Drawing for the job (mm, zero at the part's lowest x, y, z). Round coordinates to 2 decimals unless told otherwise and drop trailing zeros. Order: outer loops, then holes, each group sorted by start corner. A loop starts at its lowest first (then second) coordinate and runs counter-clockwise, first axis right, second up. Notation, with made-up numbers: (22.25, 33) -> (36.25, 33) arc R3 cw to (36.25, 37) -> close; hole circle Ø2 at (-23.75, -30). An arc over 180 degrees is marked (long way). Answer as CSV lines item,"result". Start each with the question number.
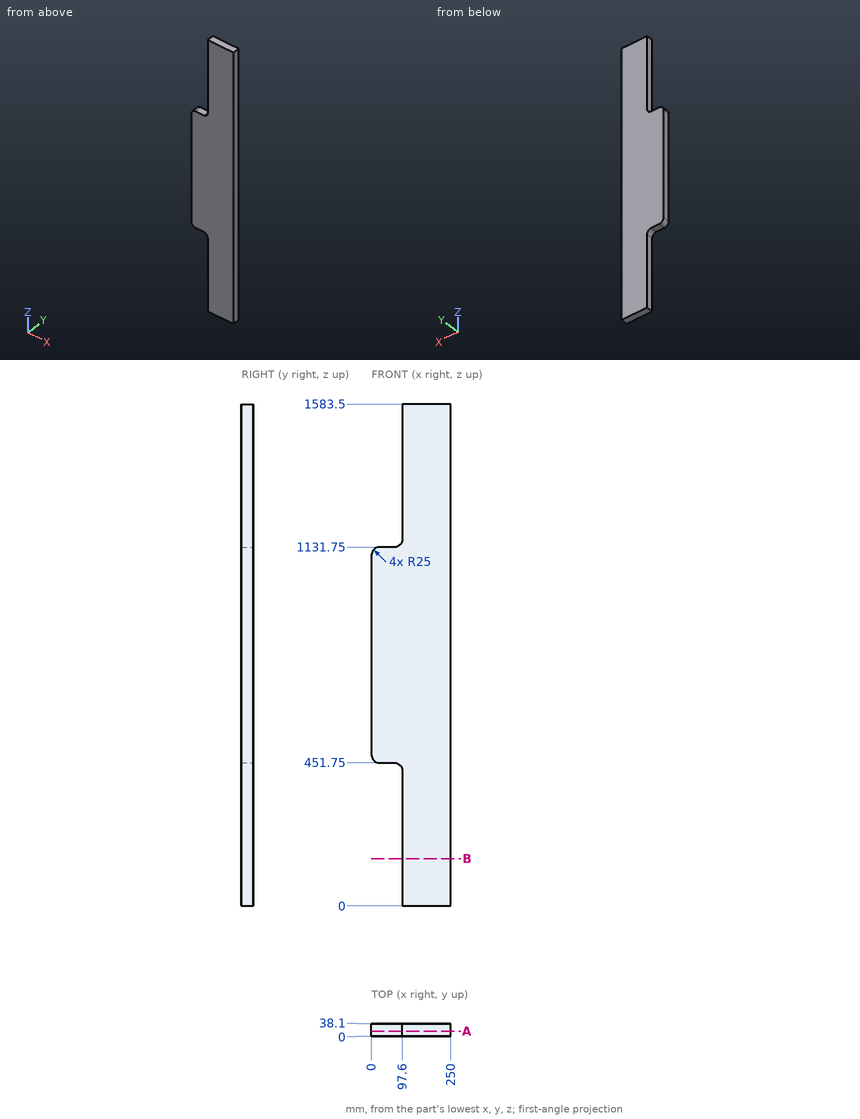
Q1. Flat gauge pins, fed straight in: pin 1 Ø5 at (x, y) = (72, 31.5) entering from +Z; pin 2 Ø8 at (y, z) = (31, 1341.5) entering from -X. Where does each tip first touch, or does it go through?
Q2. Slice it at A-A, the plane y = 15. Write the cut outline in (x, z), plus the area to 3 significant figures.
Q3. Slice it at B-B, the plane z = 149. Write the cut outline in (x, y).
Q4. Probe L1, parallel to X at y = 22, z = 324.5; L2, parallel to Z at x = 65, y = 7.5; L3, parallel to X at y = 8.5, z = 472.5. List the from-to ranges inside material, lowest first.
Solutions:
1,pin 1,"stops at z = 1131.82"
1,pin 2,"stops at x = 97.6"
2,outline,"(0, 476.75) arc R25 ccw to (25, 451.75) -> (72.6, 451.75) arc R25 cw to (97.6, 426.75) -> (97.6, 0) -> (250, 0) -> (250, 1583.5) -> (97.6, 1583.5) -> (97.6, 1156.75) arc R25 cw to (72.6, 1131.75) -> (25, 1131.75) arc R25 ccw to (0, 1106.75) -> close"
2,area,"308,000 mm2"
3,outline,"(97.6, 0) -> (250, 0) -> (250, 38.1) -> (97.6, 38.1) -> close"
4,L1,"x = 97.6 to 250"
4,L2,"z = 451.75 to 1131.75"
4,L3,"x = 0.36 to 250"
